```python
from build123d import *

# Parameters (mm, degrees)
BOSS_EXTRUDE2_DEPTH = 115
CUT_EXTRUDE1_DEPTH  = 2


with BuildPart() as part:
    # Sketch1 → Boss-Extrude2 (new body)
    with BuildSketch(Plane(origin=(0, 0, 0), x_dir=(1, 0, 0), z_dir=(0, 1, 0))):
        with BuildLine():
            Line((-98.788631121, 34.808160187), (-98.788631121, 29.808160187))
            ThreePointArc((-98.788631121, 29.808160187), (-98.202844683, 28.393946625), (-96.788631121, 27.808160187))
            Line((-96.788631121, 27.808160187), (-83.788631121, 27.808160187))
            Line((-83.788631121, 27.808160187), (-83.788631121, 18.808160187))
            Line((-83.788631121, 18.808160187), (66.211368879, 18.808160187))
            Line((66.211368879, 18.808160187), (66.211368879, 27.808160187))
            Line((66.211368879, 27.808160187), (79.211368879, 27.808160187))
            ThreePointArc((79.211368879, 27.808160187), (80.625582441, 28.393946625), (81.211368879, 29.808160187))
            Line((81.211368879, 29.808160187), (81.211368879, 34.808160187))
            ThreePointArc((81.211368879, 34.808160187), (80.625582441, 36.222373749), (79.211368879, 36.808160187))
            Line((79.211368879, 36.808160187), (-96.788631121, 36.808160187))
            ThreePointArc((-96.788631121, 36.808160187), (-98.202844683, 36.222373749), (-98.788631121, 34.808160187))
        make_face()
    extrude(amount=BOSS_EXTRUDE2_DEPTH)

    # Sketch2 → Cut-Extrude1 (cut)
    with BuildSketch(Plane(origin=(0, 0, -36.808160187), x_dir=(-1, 0, 0), z_dir=(0, 0, -1))):
        Polygon((27.408337163, 82.886030919), (3.413870614, 82.886030919), (20.114019332, 66.1858822), (9.364498318, 55.436361186), (33.071031269, 31.729828236), (-3.617725634, 55.436361186), (7.780473372, 66.1858822), (-18.469082879, 94.019463397), (27.408337163, 92.675773271), (31.055496079, 86.533189834), align=None)
    extrude(amount=-CUT_EXTRUDE1_DEPTH, mode=Mode.SUBTRACT)


solid = part.part
```
Verification items for the finished model (mm, model axes). A direction names the side the tool comes from. Coordinates: 2 decimals unless noted, no trailing zeros. Order: outer loops, then holes, each group sorted by start corner. A loop starts at its lowest first (then second) coordinate and runs counter-clockwise, first axis right, second up. Notation, with made-up numbers: (18, 74.25) -> (25, 74.25) arc R24 cw to (25, 112.25) -> close; hole circle Ø1 at (54.25, 68.25). An arc over 180 degrees is marked (long way). Answer as CSV lines item,"result". Start each with the question number.
1) Cross-section at D-D, the plane y = 64. Record the boundary of the cut face in (x, z).
2) Gauge pin test, flat ends, axial feed: pin 1 Ø4 at (x, y) = (75, 74) entering from +Z; pin 2 Ø8 at (y, z) = (42.5, -22) entering from +X; pin 3 Ø10 at (y, z) = (82, -24.5) entering from -X. Record the tip position at first contact, or that the pin passes through.
3) Cross-section at C-C, the plane z = -21.75. Record the boundary of the cut face in (x, y).
4) Set-up check for faces 1 (the face through (73, 57, -27.808)), 2 (the face through (5.16, 79.91, -35.82)), 3 (the face through (-8, 44, -36.808)): record each of +Z, -Z, +X, -X, +Y, -Y from which the full face is reachable in a straight line by a thin tool's end or side.
5) Material ranges on L1, parallel to X at y = 104, z = -26.75; L2, parallel to Z at x = -18, y = 92; L3, parallel to X at y = 39, z = -35, recorded low to high. Write a range as [from, to].
6) Release check for a two-part mould opening along Y. For faces 4 (the face through (-83.789, 57, -23)), 5 (the face through (-10, 115, -28)), 6 (the face through (-14.815, 60.886, -35.822)) record: released by +Y, released by -Y, zero draft, split by the parting line, or undercut.
7) Cross-section at B-B, the plane x = -12. Record the boundary of the cut face in (y, z).
8) Cross-section at A-A, the plane y = 21. Record the boundary of the cut face in (x, z), then the cut area to 3 significant figures.
Conclusion:
1,outline,"(-98.79, -34.81) arc R2 ccw to (-96.79, -36.81) -> (-17.93, -36.81) -> (-17.93, -34.81) -> (-5.46, -34.81) -> (-5.46, -36.81) -> (79.21, -36.81) arc R2 ccw to (81.21, -34.81) -> (81.21, -29.81) arc R2 ccw to (79.21, -27.81) -> (66.21, -27.81) -> (66.21, -18.81) -> (-83.79, -18.81) -> (-83.79, -27.81) -> (-96.79, -27.81) arc R2 ccw to (-98.79, -29.81) -> close"
2,pin 1,"stops at z = -27.81"
2,pin 2,"stops at x = 66.21"
2,pin 3,"stops at x = -98.76"
3,outline,"(-83.79, 0) -> (66.21, 0) -> (66.21, 115) -> (-83.79, 115) -> close"
4,face 1,"+Z, +X, +Y, -Y"
4,face 2,"-Z"
4,face 3,"-Z, +X, -X, +Y, -Y"
5,L1,"x = [-83.79, 66.21]"
5,L2,"z = [-34.81, -18.81]"
5,L3,"x = [-98.78, -25.8], [-21.82, 81.2]"
6,face 4,"zero draft"
6,face 5,"released by +Y"
6,face 6,"undercut"
7,outline,"(0, -36.81) -> (45.34, -36.81) -> (45.34, -34.81) -> (52.8, -34.81) -> (52.8, -36.81) -> (58.07, -36.81) -> (58.07, -34.81) -> (74.3, -34.81) -> (74.3, -36.81) -> (82.89, -36.81) -> (82.89, -34.81) -> (93.13, -34.81) -> (93.13, -36.81) -> (115, -36.81) -> (115, -18.81) -> (0, -18.81) -> close"
8,outline,"(-98.79, -34.81) arc R2 ccw to (-96.79, -36.81) -> (79.21, -36.81) arc R2 ccw to (81.21, -34.81) -> (81.21, -29.81) arc R2 ccw to (79.21, -27.81) -> (66.21, -27.81) -> (66.21, -18.81) -> (-83.79, -18.81) -> (-83.79, -27.81) -> (-96.79, -27.81) arc R2 ccw to (-98.79, -29.81) -> close"
8,area,"2,970 mm²"
